```python
from build123d import *

# Parameters (mm, degrees)
ZAOKR_GLENIE1_R             = 0.2
SZKIC3_R                    = 3
DODANIE_WYCI_GNI_CIE1_DEPTH = 10


with BuildPart() as part:
    # Szkic1 → Obrót1 (revolve)
    with BuildSketch(Plane.XY):
        Polygon((0, 2), (152, 2), (152, 6.45), (144, 6.45), (144, 8.25), (125, 8.25), (125, 6.45), (0, 6.45), align=None)
    revolve(axis=Axis((0, 0, 0), (1, 0, 0)))

    # Zaokrąglenie1
    zaokr_glenie1_edges = [part.edges().sort_by_distance(p)[0] for p in [
        (152, -6.45, 0),
        (144, -8.25, 0),
        (125, -8.25, 0),
        (0, -6.45, 0),
    ]]
    fillet(zaokr_glenie1_edges, radius=ZAOKR_GLENIE1_R)

    # Szkic3 → Dodanie-wyciągnięcie1 (add)
    with BuildSketch(Plane(origin=(0, 0, 2), x_dir=(-1, 0, 0), z_dir=(0, 0, -1))):
        with Locations((-138, 0)):
            Circle(SZKIC3_R)
    extrude(amount=-DODANIE_WYCI_GNI_CIE1_DEPTH)


solid = part.part
```
Build history of the part. All positions in model axes, mm. A direction names the side the tool comes from. Round coordinates to 2 decimals unless told otherwise and drop trailing zeros. Order: outer loops, then holes, each group sorted by start corner. A loop starts at its lowest first (then second) coordinate and runs counter-clockwise, first axis right, second up. Notation, with made-up numbers: (-37.75, 26.5) -> (-30.75, 26.5) arc R18 ccw to (-30.75, 39.5) -> close; hole circle Ø5 at (70, 86). An arc over 180 degrees is marked (long way). Answer in a Markdown table with one row per item.
1) Band-saw the part on D-D on x = 82. Give the cut face in (y, z), and give its area (3 significant figures).
Values:
| item | result |
|---|---|
| outline | circle Ø12.9 at (0, 0); hole circle Ø4 at (0, 0) |
| area | 118 mm2 |
2) Band-saw the part on B-B on y = 0. Give the cut face in (x, z), and give its area (3 significant figures).
Values:
| item | result |
|---|---|
| outline | (0, -6.25) arc R0.2 ccw to (0.2, -6.45) -> (125, -6.45) -> (125, -8.05) arc R0.2 ccw to (125.2, -8.25) -> (143.8, -8.25) arc R0.2 ccw to (144, -8.05) -> (144, -6.45) -> (151.8, -6.45) arc R0.2 ccw to (152, -6.25) -> (152, -2) -> (0, -2) -> close; (0, 2) -> (152, 2) -> (152, 6.25) arc R0.2 ccw to (151.8, 6.45) -> (144, 6.45) -> (144, 8.05) arc R0.2 ccw to (143.8, 8.25) -> (141, 8.25) -> (141, 12) -> (135, 12) -> (135, 8.25) -> (125.2, 8.25) arc R0.2 ccw to (125, 8.05) -> (125, 6.45) -> (0.2, 6.45) arc R0.2 ccw to (0, 6.25) -> close |
| area | 1,440 mm2 |
3) Pin check, flat tips, straight feed: P1, Ø5, axis at x = 15.5, z = 5, coming from the -Y side; P2, Ø5, axis at x = 68.5, z = -5.5, coming from the -Y side; P3, Ø4, axis at x = 95, z = 9.5, coming from the +Y side; P4, Ø10, axis at x = 69.5, z = 1.5, coming from the -Y side. Stop position of each tip, or through.
Values:
| item | result |
|---|---|
| P1 | y = -5.95 |
| P2 | y = -5.71 |
| P3 | through |
| P4 | y = -6.45 |
4) Mould opens along Z. For faces 4 (the cylindrical face through (135.14, 0.9, 9.81)), 5 (the cylindrical face through (77, 0, -2)), 6 (the cylindrical face through (61.726, -1.398, -6.297)) say: released by +Z, released by -Z, zero draft, split by the parting line, or undercut.
Values:
| item | result |
|---|---|
| face 4 | zero draft |
| face 5 | undercut |
| face 6 | split by the parting line |
5) Which spindle directions (+Z, -Z, +X, -X, +Y, -Y) get a long thin tool onto all of the face, cutting with end or side? Do faces 1 (the cylindrical face through (147.845, -1.398, -6.297)), 2 (the flat face through (125, 0, 7)), 3 (the flat face through (152, 0, -3)). Say none if no direction does.
Values:
| item | result |
|---|---|
| face 1 | +X |
| face 2 | -X |
| face 3 | +Z, -Z, +X, +Y, -Y |
6) Band-saw the part on C-C on x = 138. Give the cut face in (y, z), and give its area (3 significant figures).
Values:
| item | result |
|---|---|
| outline | (-3, 7.69) arc R8.25 ccw (long way) to (3, 7.69) -> (3, 12) -> (-3, 12) -> close; hole circle Ø4 at (0, 0) |
| area | 225 mm2 |
7) Wall check: L1, parallel to Z at x = 114, y = 0; L2, parallel to X at y = 6, z = 3.25; L3, parallel to Z at x = 89, y = -0.75. Give the ranges that are in metal, low to high.
Values:
| item | result |
|---|---|
| L1 | -6.45 to -2, 2 to 6.45 |
| L2 | 125 to 144 |
| L3 | -6.41 to -1.85, 1.85 to 6.41 |
8) Band-saw the part on A-A on z = 0. Give the cut face in (x, y).
Values:
| item | result |
|---|---|
| outline | (0, -6.25) arc R0.2 ccw to (0.2, -6.45) -> (125, -6.45) -> (125, -8.05) arc R0.2 ccw to (125.2, -8.25) -> (143.8, -8.25) arc R0.2 ccw to (144, -8.05) -> (144, -6.45) -> (151.8, -6.45) arc R0.2 ccw to (152, -6.25) -> (152, -2) -> (0, -2) -> close; (0, 2) -> (152, 2) -> (152, 6.25) arc R0.2 ccw to (151.8, 6.45) -> (144, 6.45) -> (144, 8.05) arc R0.2 ccw to (143.8, 8.25) -> (125.2, 8.25) arc R0.2 ccw to (125, 8.05) -> (125, 6.45) -> (0.2, 6.45) arc R0.2 ccw to (0, 6.25) -> close |
